Drawing for the job (mm, zero at the part's lowest x, y, z). A direction names the side the tool comes from. Coordinates: 2 decimals unless noted, no trailing zeros. Write each loop counter-clockwise with the first axis right and the second up, starting at its lowest first coordinate (ties: lowest second). Pieces come first, ordered by that corner, then holes. Notation, with made-up numbers: (64, 60) -> (77, 60) arc R20 cw to (77, 81) -> close; hole circle Ø6 at (82, 5). An arc over 180 degrees is marked (long way). Write each question's results on one line, items separated by ' | '. Start each with the question number.
Q1. Drill centre lines: line 1 (Z direction, x = 29, y = 26); line 2 (Z direction, x = 14.5, y = 21.5); line 3 (Y direction, x = 18.5, z = 40). Where is each one in solid material? Low to high.
Q2. Saw through at A-A on y = 19.25. Give the cut face in (x, z), and give its area (3 significant figures).
Q3. Drop flat-ended pins along their axis: pin 1 Ø4 at (x, z) = (27, 14) entering from -Y; pin 2 Ø2 at (x, z) = (6.5, 45.5) entering from -Y; pin 3 Ø12 at (x, z) = (19.5, 26) entering from +Y; pin 4 Ø10 at (y, z) = (5, 8.5) entering from +X. Give the stop position or say it passes through.
Q4. Saw through at D-D on z = 7.5. Give the cut face in (x, y).
Q5. Saw through at C-C on z = 27.5. Give the cut face in (x, y), and give its area (3 significant figures).
Q6. Tool access for the marked faces 1 and 2: list every direction of +Z, -Z, +X, -X, +Y, -Y with a clear straight run to the whole face (end or side of a thin tool).
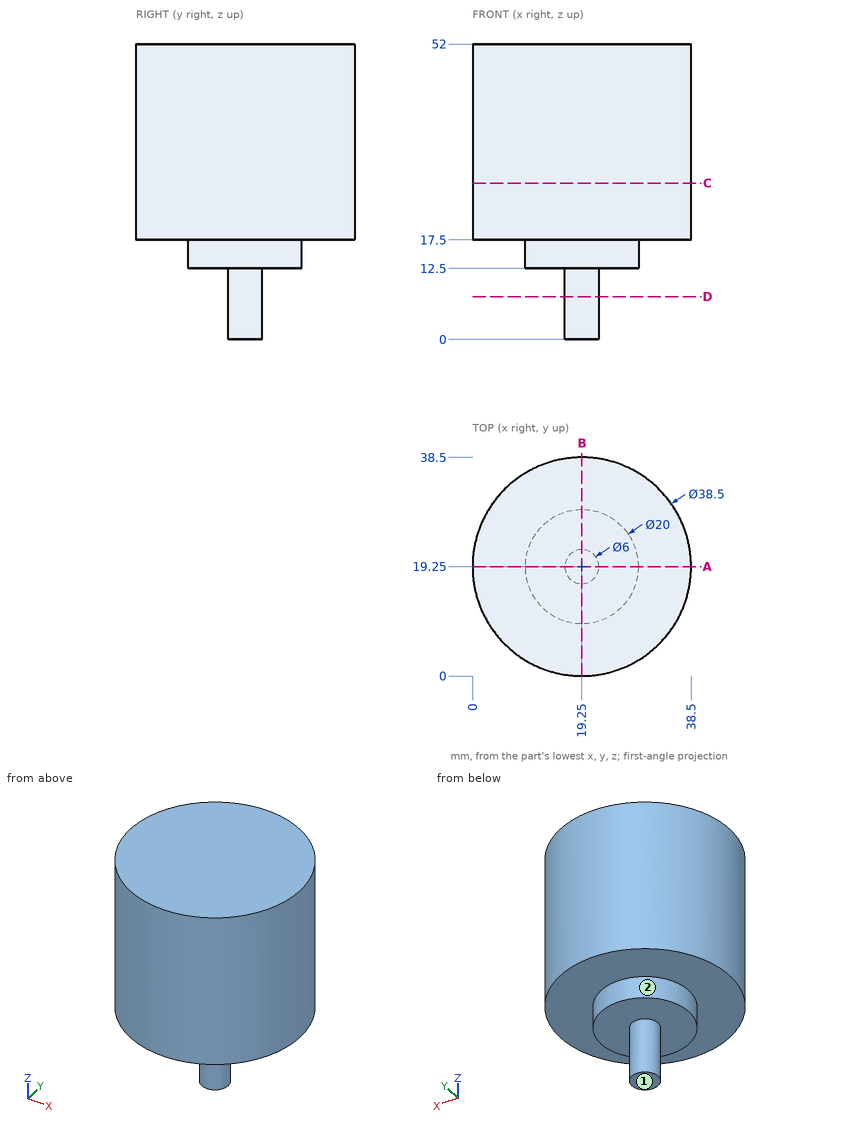
Returned:
1) line 1: z = 17.5 to 52 | line 2: z = 12.5 to 52 | line 3: y = 0.01 to 38.49
2) outline: (0, 17.5) -> (9.25, 17.5) -> (9.25, 12.5) -> (16.25, 12.5) -> (16.25, 0) -> (22.25, 0) -> (22.25, 12.5) -> (29.25, 12.5) -> (29.25, 17.5) -> (38.5, 17.5) -> (38.5, 52) -> (0, 52) -> close | area: 1,500 mm2
3) pin 1: stops at y = 11.07 | pin 2: stops at y = 4 | pin 3: stops at y = 38.5 | pin 4: passes through
4) outline: circle Ø6 at (19.25, 19.25)
5) outline: circle Ø38.5 at (19.25, 19.25) | area: 1,160 mm2
6) face 1: -Z, +X, -X, +Y, -Y | face 2: -Z
